Autodesk Inventor part; units mm, degrees
ref_plane "YZ Plane" through (0, 0, 0) normal (1, 0, 0) x (0, 1, 0)
ref_plane "XZ Plane" through (0, 0, 0) normal (0, 1, 0) x (-1, 0, 0)
ref_plane "XY Plane" through (0, 0, 0) normal (0, 0, 1) x (1, 0, 0)
sketch "スケッチ1" plane through (0, 0, 0) normal (0, 0, 1) x (1, 0, 0)
  circle A0 centre (0, 0) radius 20
  dimension "d0" = 40
extrude "押し出し1" add sketch "スケッチ1" along normal blind 8
sketch "スケッチ2" plane through (0, 0, 8) normal (0, 0, 1) x (1, 0, 0)
  circle A0 centre (0, 0) radius 16
  point P0 (0, 16)
  point P1 (-13.8564, 8)
  point P2 (-13.8564, -8)
  point P3 (0, -16)
  point P4 (13.8564, -8)
  point P5 (13.8564, 8)
  dimension "d3" = 32
  dimension "d6" = 360
hole "穴1" at (0, 16, 8) at (-13.8564, 8, 8) at (-13.8564, -8, 8) at (0, -16, 8) at (13.8564, -8, 8) at (13.8564, 8, 8) direction (0, 0, -1) diameter 3.2 end through all
sketch "スケッチ3" plane through (0, 0, 0) normal (0, 0, -1) x (-1, 0, 0)
  circle A0 centre (0, 0) radius 9
  point P0 (0, 9)
  point P1 (-9, 0)
  point P2 (0, -9)
  point P3 (9, 0)
  dimension "d15" = 18
  dimension "d18" = 360
hole "穴2" at (0, 9, 0) at (9, 0, 0) at (0, -9, 0) at (-9, 0, 0) direction (0, 0, 1) diameter 4.3 end through all
sketch "スケッチ4" plane through (0, 0, 8) normal (0, 0, 1) x (1, 0, 0)
  circle A0 centre (0, 0) radius 4.1
  dimension "d27" = 8.2
extrude "押し出し2" cut sketch "スケッチ4" against normal blind 6
sketch "スケッチ5" plane through (0, 0, 8) normal (0, 0, 1) x (1, 0, 0)
  line L0 (-14, -14) -> (14, -14)
  line L1 (14, -14) -> (14, 14)
  line L2 (14, 14) -> (-14, 14)
  line L3 (-14, 14) -> (-14, -14)
  line L4 (-14, -14) -> (14, 14) construction
  line L5 (14, -14) -> (-14, 14) construction
  point P0 (0, 0)
  dimension "d30" = 28
  dimension "d31" = 28
hole "穴3" at (-14, 14, 8) at (14, 14, 8) at (14, -14, 8) at (-14, -14, 8) direction (0, 0, -1) diameter 2.2 end through all counterbore diameter 4.4 counterbore depth 20
fillet "フィレット1" radius 1 8 edges at (15.611, -12.5018, 4) (15.611, 12.5018, 4) (12.5018, 15.611, 4) (12.5018, -15.611, 4) (-12.5018, -15.611, 4) (-15.611, -12.5018, 4) (-15.611, 12.5018, 4) (-12.5018, 15.611, 4)
properties part number "scara-base18" material "ABS プラスチック"
CAD build for the part. Positions are in the model's coordinates, mm. A direction names the side the tool comes from. Give positions to 0.01 mm unless a question says otherwise; leave off trailing zeros. Order: outer loops, then holes, each group sorted by start corner. A loop starts at its lowest first (then second) coordinate and runs counter-clockwise, first axis right, second up. Notation, with made-up numbers: (73, 76) -> (129, 76) arc R29 cw to (129, 107) -> close; hole circle Ø3 at (28.5, 23). An arc over 180 degrees is marked (long way). Return JSON: item names as keys, results as strings.
Q1. Mould opens along X. For faces 1 (the face through (-20, 0, 4)), 2 (the face through (12.47, 12.42, 3.94)), 3 (the face through (0, 5, 8)), 4 (the face through (12.8, -6.8, 3.9)) say: pulls with the +X half, pulls with the -X half, needs draft (parallel to the pull), parting line crosses it, or undercut.
Working result:
{"face 1": "pulls with the -X half", "face 2": "undercut", "face 3": "needs draft", "face 4": "undercut"}
Q2. Saw through at C-C (x = 9). Write the cut outline in (y, z), then the cut area to 3 significant figures.
Working result:
{"outline": "(-17.86, 0) -> (-2.15, 0) -> (-2.15, 8) -> (-17.86, 8) -> close; (2.15, 0) -> (17.86, 0) -> (17.86, 8) -> (2.15, 8) -> close", "area": "251 mm²"}
Q3. Which spindle directions (+Z, -Z, +X, -X, +Y, -Y) get a long thin tool onto all of the face, cutting with end or side? Do faces 5 (the face through (-0.09, -11.15, 4.06)), 6 (the face through (0, 0, 2)). Say none if no direction does.
Working result:
{"face 5": "+Z, -Z", "face 6": "+Z"}
Q4. Saw through at D-D (z = 5). Count the separate pieces of the cut face and the enclosed holes in it, then the cut area to 3 significant figures.
Working result:
{"separate pieces": "1", "enclosed holes": "11", "area": "1,060 mm²"}
Q5. Saw through at B-B (y = 8). Write the cut outline in (x, z), then the cut area to 3 significant figures.
Working result:
{"outline": "(-18.33, 0) -> (-15.46, 0) -> (-15.46, 8) -> (-18.33, 8) -> close; (-12.26, 0) -> (-1.9, 0) -> (-1.9, 8) -> (-12.26, 8) -> close; (1.9, 0) -> (12.26, 0) -> (12.26, 8) -> (1.9, 8) -> close; (15.46, 0) -> (18.33, 0) -> (18.33, 8) -> (15.46, 8) -> close", "area": "212 mm²"}
Q6. Flat gauge pins, fed straight in: pin 1 (3 mm diameter, centred on x = 13.86, y = -8, fed in from -Z); pin 2 (4 mm diameter, centred on x = 11, z = 4.5, fed in from +Y); pin 3 (2 mm diameter, centred on x = 14, z = 4.5, fed in from -Y); pin 4 (7.5 mm diameter, centred on x = 0, y = 0, fed in from +Z). Where does each tip first touch, or does it go through?
Working result:
{"pin 1": "through", "pin 2": "y = 17.86", "pin 3": "y = -12.04", "pin 4": "z = 2"}
Q7. Drill centre lines: line 1 (Y direction, x = -1, z = 6.5); line 2 (X direction, y = 8, z = 5.5); line 3 (X direction, y = 10, z = 3.75). Where is each one in solid material? Low to high.
Working result:
{"line 1": "-19.97 to -17.25, -14.75 to -10.9, -7.1 to -3.98, 3.98 to 7.1, 10.9 to 14.75, 17.25 to 19.97", "line 2": "-18.33 to -15.46, -12.26 to -1.9, 1.9 to 12.26, 15.46 to 18.33", "line 3": "-17.32 to -1.9, 1.9 to 17.32"}
Q8. Saw through at A-A (y = 0). Write the cut outline in (x, z), then the cut area to 3 significant figures.
Working result:
{"outline": "(-20, 0) -> (-11.15, 0) -> (-11.15, 8) -> (-20, 8) -> close; (-6.85, 0) -> (6.85, 0) -> (6.85, 8) -> (4.1, 8) -> (4.1, 2) -> (-4.1, 2) -> (-4.1, 8) -> (-6.85, 8) -> close; (11.15, 0) -> (20, 0) -> (20, 8) -> (11.15, 8) -> close", "area": "202 mm²"}
